```python
from build123d import *

# Parameters (mm, degrees)
EXTRUDE_THIN1_DEPTH = 889
SKETCH5_W           = 304.838367632
SKETCH5_H           = 889
CUT_EXTRUDE1_DEPTH  = 1035.425821721


with BuildPart() as part:
    # Sketch2 → Extrude-Thin1 (new body)
    with BuildSketch(Plane.XY):
        with BuildLine():
            Line((-156.728695436, -203.89972205), (150.180738454, -208.769553389))
            ThreePointArc((150.180738454, -208.769553389), (4.080165374, 257.142631385), (-156.728695436, -203.89972205))
        make_face()
        with BuildLine():
            Line((-155.623606079, -200.741857197), (149.176393921, -205.578217466))
            ThreePointArc((149.176393921, -205.578217466), (4.029792962, 253.968030997), (-155.623606079, -200.741857197))
        make_face(mode=Mode.SUBTRACT)
    extrude(amount=EXTRUDE_THIN1_DEPTH)

    # Sketch5 → Cut-Extrude1 (cut, through all)
    with BuildSketch(Plane(origin=(-3.223606079, -203.160037332, 0), x_dir=(0.9998741377849476, -0.01586532662152281, 0), z_dir=(0.01586532662152281, 0.9998741377849476, 0))):
        with Locations((0, -444.5)):
            Rectangle(SKETCH5_W, SKETCH5_H)
    extrude(amount=-CUT_EXTRUDE1_DEPTH, mode=Mode.SUBTRACT)


solid = part.part
```
Design review of the part built by this model. Coordinates are the model's own, in mm. Give positions to 0.01 mm unless a question says otherwise; leave off trailing zeros. Order: outer loops, then holes, each group sorted by start corner. A loop starts at its lowest first (then second) coordinate and runs counter-clockwise, first axis right, second up. Notation, with made-up numbers: (59.5, 25) -> (110.5, 25) arc R21 cw to (110.5, 51) -> close; hole circle Ø10 at (-36.75, 6). An arc over 180 degrees is marked (long way). Write item = value, one per line. Start each with the question number.
(1) We need section C-C on z = 273. Write out the cut boundary in (x, y) (3 decimals).
(2) To check wall thickness, follow line 1 along X through (y, z) = (0, 324.5) (3 decimals); line 2 along X through (y, z) = (6.5, 141); line 3 along Y through (x, z) = (0, 210) (3 decimals). State the ranges of each line that lie inside material, in increasing order.
(3) For pin 1 (2 mm diameter, centred on x = 29, z = 352.5, fed in from -Y); pin 2 (3 mm diameter, centred on y = -64.5, z = 616, fed in from +X); pin 3 (8 mm diameter, centred on y = -107, z = 632, fed in from +X), all flat-tipped, find the tip position at first contact; note any pin that passes through.
(4) We need section A-A on y = 0. Write out the cut boundary in (x, z) (3 decimals), plus the area to 3 significant figures.
(5) We need section D-D on x = 0. Write out the cut boundary in (y, z) (3 decimals).
(6) Mouldability with a two-part tool opening along Y and no side actions: class faces 1 (the face through (12.91, 253.67, 438.28)), 2 (the face through (13.083, 256.842, 438.277)) as +Y half, -Y half, draft (parallel to the pull), parting line (faces both ways), or undercut.
(7) We need section B-B on x = 169. Write out the cut boundary in (y, z).
Numbers:
q1.outline = (-156.729, -203.9) -> (-155.674, -203.916) -> (-155.624, -200.742) arc R254 cw (long way) to (149.176, -205.578) -> (149.126, -208.753) -> (150.181, -208.77) arc R257.175 ccw (long way) to start
q2.line_1 = -257.175 to -254, 254 to 257.175
q2.line_2 = -257.09 to -253.92, 253.92 to 257.09
q2.line_3 = 254 to 257.175
q3.pin_1 = 252.22
q3.pin_2 = 249.34
q3.pin_3 = 235.65
q4.outline = (-257.175, 0) -> (-254, 0) -> (-254, 889) -> (-257.175, 889) -> close; (254, 0) -> (257.175, 0) -> (257.175, 889) -> (254, 889) -> close
q4.area = 5,650 mm^2
q5.outline = (254, 0) -> (257.175, 0) -> (257.175, 889) -> (254, 889) -> close
q6.face_1 = undercut
q6.face_2 = parting line
q7.outline = (-193.85, 0) -> (-189.62, 0) -> (-189.62, 889) -> (-193.85, 889) -> close; (189.62, 0) -> (193.85, 0) -> (193.85, 889) -> (189.62, 889) -> close
